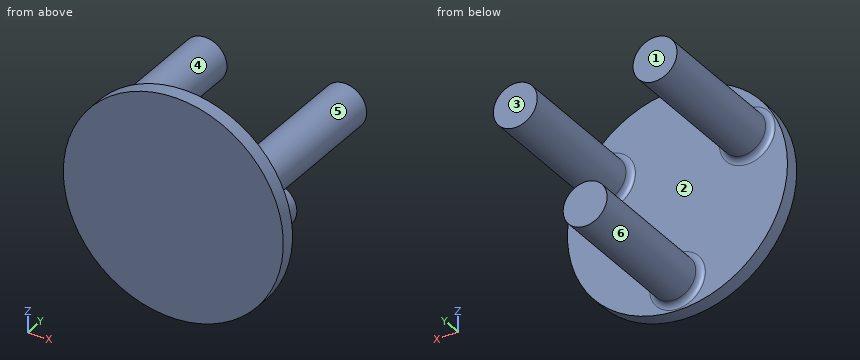
Autodesk Inventor part; units mm, degrees
ref_plane "YZ Plane" through (0, 0, 0) normal (1, 0, 0) x (0, 1, 0)
ref_plane "XZ Plane" through (0, 0, 0) normal (0, 1, 0) x (-1, 0, 0)
ref_plane "XY Plane" through (0, 0, 0) normal (0, 0, 1) x (1, 0, 0)
sketch "スケッチ1" plane through (0, 0, 0) normal (0, 1, 0) x (-1, 0, 0)
  circle A0 centre (0, 0) radius 75
  dimension "d0" = 150
extrude "押し出し1" add sketch "スケッチ1" along normal blind 10
sketch "スケッチ2" plane through (0, 10, 0) normal (0, 1, 0) x (1, 0, 0)
  circle A0 centre (0, 55) radius 15
  circle A1 centre (-47.6314, -27.5) radius 15
  circle A2 centre (47.6314, -27.5) radius 15
  point P0 (0, 0)
  dimension "d3" = 30
  dimension "d4" = 55
  dimension "d7" = 360
extrude "押し出し2" add sketch "スケッチ2" along normal blind 100
fillet "フィレット1" radius 4 3 edges at (-62.6314, 10, 27.5) (32.6314, 10, 27.5) (-15, 10, -55)
Design review of the part built by this model. Coordinates are the model's own, in mm. Face numbers are marked on the shaded views. A direction names the side the tool comes from. Round coordinates to 2 decimals unless told otherwise and drop trailing zeros. Write each loop counter-clockwise with the first axis right and the second up, starting at its lowest first coordinate (ties: lowest second). Pieces come first, ordered by that corner, then holes. Notation, with made-up numbers: (53.25, -36) -> (71.25, -36) arc R18 ccw to (71.25, -13) -> close; hole circle Ø6 at (10, 3). An arc over 180 degrees is marked (long way). One line per item, written item: value. Start each with the question number.
Q1. Add section A-A (x = 0). Give the boundary of the cut face in (y, z).
Q2. Insertion check: P1, Ø3, axis at x = -35, z = -55.5, coming from the +Y side; P2, Ø4, axis at x = -52, y = 82, coming from the -Z side; P3, Ø1, axis at x = 5.5, z = -44.5, coming from the -Y side; P4, Ø5, axis at x = -14, y = 79, coming from the +Z side. Each pin has a flat end and moves straight along its axis. Give the tip position at first contact, or say it passes through.
Q3. To check wall thickness, follow probe 1 along Y at (x, z) = (5, -11); probe 2 along X at (y, z) = (14, 15); probe 3 along Z at (x, y) = (-34, 20). State the ranges of each line that lie inside material, in increasing order.
Q4. Tool access review of the marked faces 1 and 2: name each direction out of +Z, -Z, +X, -X, +Y, -Y from which nothing blocks a thin tool from reaching the whole face with its end or side.
Q5. Add section C-C (z = -55). Give the boundary of the cut face in (x, y), then the cut area to 3 significant figures.
Q6. Add section B-B (y = 40). Give the boundary of the cut face in (x, z).
Q7. Add section D-D (y = 7.5). Give the boundary of the cut face in (x, z).
Q8. The part is to be moulded in two halves that separate along X. For the marked faces 3, 4, 5 and 6, say which applies: pulls with the +X half, pulls with the -X half, needs draft (parallel to the pull), parting line crosses it, or undercut.
Response:
1. outline: (0, -75) -> (10, -75) -> (10, -74) arc R4 cw to (14, -70) -> (110, -70) -> (110, -40) -> (14, -40) arc R4 cw to (10, -36) -> (10, 75) -> (0, 75) -> close
2. P1: stops at y = 10
2. P2: stops at z = 12.69
2. P3: stops at y = 0
2. P4: stops at z = -45.37
3. probe 1: y = 0 to 10
3. probe 2: x = -55.92 to -39.34, 39.34 to 55.92
3. probe 3: z = 21.24 to 33.76
4. face 1: +Z, -Z, +X, -X, +Y
4. face 2: +Y
5. outline: (-50.99, 0) -> (50.99, 0) -> (50.99, 10) -> (19, 10) arc R4 cw to (15, 14) -> (15, 110) -> (-15, 110) -> (-15, 14) arc R4 cw to (-19, 10) -> (-50.99, 10) -> close
5. area: 4,030 mm^2
6. outline: circle Ø30 at (-47.63, 27.5); circle Ø30 at (0, -55); circle Ø30 at (47.63, 27.5)
7. outline: circle Ø150 at (0, 0)
8. face 3: needs draft
8. face 4: undercut
8. face 5: undercut
8. face 6: parting line crosses it
